Build history of the part. All positions in model axes, mm. A direction names the side the tool comes from. Round coordinates to 2 decimals unless told otherwise and drop trailing zeros. Loops run counter-clockwise (first coordinate to the right, second up) from the corner with the lowest first, then second, coordinate; pieces in that order, holes last. Notation, with made-up numbers: M -17.75,60 L 37.25,60 A22 cw 37.25,89 Z; hole C 74,-35.5 d2. An arc over 180 degrees is marked long. Write each question's results on one line, items separated by ' | '. Start each with the question number.
```python
from build123d import *

# Parameters (mm, degrees)
SKETCH_1_W          = 16
SKETCH_1_H          = 6
SKETCH_1_R          = 1.5
EXTRUDE_1_DEPTH     = 5
SKETCH_2_W          = 16
SKETCH_2_H          = 70
EXTRUDE_2_DEPTH     = 4
SKETCH_3_R          = 2
CUT_EXTRUDE_1_DEPTH = 72.414284285
SKETCH_4_R          = 2
CUT_EXTRUDE_2_DEPTH = 72.414284285
SKETCH_5_R          = 3.5
CUT_EXTRUDE_3_DEPTH = 0.8
EXTRUDE_3_DEPTH     = 3
FILLET_1_R          = 10


with BuildPart() as part:
    # 草图1 → 凸台-拉伸1 (new body)
    with BuildSketch(Plane(origin=(0, 0, 0), x_dir=(1, 0, 0), z_dir=(0, 1, 0))):
        with Locations((2, 0)):
            Rectangle(SKETCH_1_W, SKETCH_1_H)
        with Locations(Location((-3, 0, 0), (0, 0, 270))):
            Circle(SKETCH_1_R, mode=Mode.SUBTRACT)
        with Locations(Location((7, 0, 0), (0, 0, 270))):
            Circle(SKETCH_1_R, mode=Mode.SUBTRACT)
    extrude(amount=EXTRUDE_1_DEPTH)

    # 草图2 → 凸台-拉伸2 (add)
    with BuildSketch(Plane(origin=(0, 0, -3), x_dir=(-1, 0, 0), z_dir=(0, 0, -1))):
        with Locations((-2, 35)):
            Rectangle(SKETCH_2_W, SKETCH_2_H)
    extrude(amount=EXTRUDE_2_DEPTH)

    # 草图3 → 切除-拉伸1 (cut, through all)
    with BuildSketch(Plane(origin=(0, 0, -7), x_dir=(-1, 0, 0), z_dir=(0, 0, -1))):
        with Locations((-5, 65)):
            Circle(SKETCH_3_R)
    extrude(amount=-CUT_EXTRUDE_1_DEPTH, mode=Mode.SUBTRACT)

    # 草图4 → 切除-拉伸2 (cut, through all)
    with BuildSketch(Plane(origin=(0, 0, -7), x_dir=(-1, 0, 0), z_dir=(0, 0, -1))):
        with Locations((0, 24.5)):
            Circle(SKETCH_4_R)
    extrude(amount=-CUT_EXTRUDE_2_DEPTH, mode=Mode.SUBTRACT)

    # 草图5 → 切除-拉伸3 (cut)
    with BuildSketch(Plane(origin=(0, 0, -7), x_dir=(-1, 0, 0), z_dir=(0, 0, -1))):
        with Locations((-5, 65)):
            Circle(SKETCH_5_R)
    extrude(amount=-CUT_EXTRUDE_3_DEPTH, mode=Mode.SUBTRACT)

    # 草图6 → 凸台-拉伸3 (add)
    with BuildSketch(Plane(origin=(10, 0, 0), x_dir=(0, 0, -1), z_dir=(1, 0, 0))):
        Polygon((3, 5), (-3, 5), (-3, 0), (7, 0), (7, 45), (3, 45), align=None)
        Polygon((3, 45), (-3, 5), (3, 5), align=None)
    extrude(amount=EXTRUDE_3_DEPTH)

    # 圆角1
    # the kernel refuses this fillet: 10 mm, written as the material it adds along each edge
    with BuildSketch(Plane(origin=(10, 45, -7), x_dir=(0, 1, 0), z_dir=(0, 0, 1))) as fillet_1_piece_1:
        with BuildLine():
            CenterArc((7.141428429, -10), FILLET_1_R, 90, 45.572995999)
            Line((0, -3), (0, 0))
            Line((0, 0), (7.141428429, 0))
        make_face()
    extrude(amount=4)


solid = part.part
```
Item 1: Tool access for faces 1 (the flat face through (10, 16, -1)), 2 (the flat face through (10, 61, -5)), 3 (the flat face through (3, 63, -6.2)): list every direction of +Z, -Z, +X, -X, +Y, -Y with a clear straight run to the whole face (end or side of a thin tool).
Item 2: Drill centre lines: line 1 along X through (y, z) = (2.5, 0); line 2 along Y through (x, z) = (0, -4.3); line 3 along Y through (x, z) = (5, -6.8). Where is each one in solid material? Low to high. Write a range as [from, to].
Item 3: Saw through at C-C, the plane y = 10. Give the cut face in (x, z).
Item 4: Saw through at B-B, the plane z = 0. Give the cut face in (x, y), then the cut area to 3 significant figures.
Item 5: Mould opens along Y. For faces 4 (the cylindrical face through (3.12, 67.95, -6.61)), 5 (the cylindrical face through (10.76, 48.32, -5.03)), 6 (the flat face through (3, 38, -3)) say: released by +Y, released by -Y, zero draft, split by the parting line, or undercut.
Item 6: Saw through at A-A, the plane x = 0. Give the cut face in (y, z), then the cut area to 3 significant figures.
Item 7: Saw through at D-D, the plane y = 24.5. Give the cut face in (x, z) (3 decimals), then the cut area to 3 significant figures.
Item 8: Drop flat-ended pins along their axis: pin 1 (6 mm diameter, centred on x = 9, z = -0.5, fed in from -Y); pin 2 (6 mm diameter, centred on x = -4, z = 0.5, fed in from +Y); pin 3 (4.5 mm diameter, centred on x = 0, y = 24.5, fed in from +Z); pin 4 (1.2 mm diameter, centred on y = 60.5, z = -5, fed in from +X). Give the stop position or say it passes through.
Working result:
1) face 1: +Z, -X, +Y | face 2: +Z, -Z, +X, +Y | face 3: -Z
2) line 1: x = [-6, -4.5], [-1.5, 5.5], [8.5, 13] | line 2: y = [0, 22.5], [26.5, 70] | line 3: y = [0, 61.5], [68.5, 70]
3) outline: M -6,-7 L 13,-7 L 13,2.25 L 10,2.25 L 10,-3 L -6,-3 Z
4) outline: M -6,0 L -4.5,0 L -4.5,5 L -6,5 Z; M -1.5,0 L 5.5,0 L 5.5,5 L -1.5,5 Z; M 8.5,0 L 13,0 L 13,25 L 10,25 L 10,5 L 8.5,5 Z | area: 125 mm²
5) face 4: undercut | face 5: released by +Y | face 6: zero draft
6) outline: M 0,-7 L 22.5,-7 L 22.5,-3 L 5,-3 L 5,3 L 0,3 Z; M 26.5,-7 L 70,-7 L 70,-3 L 26.5,-3 Z | area: 294 mm²
7) outline: M -6,-7 L -2,-7 L -2,-3 L -6,-3 Z; M 2,-7 L 13,-7 L 13,0.075 L 10,0.075 L 10,-3 L 2,-3 Z | area: 69.2 mm²
8) pin 1: stops at y = 0 | pin 2: stops at y = 5 | pin 3: stops at z = -3 | pin 4: stops at x = 10
